Model file for the job. Use its own axes, mm. Face numbers are marked on the shaded views. A direction names the side the tool comes from. Round coordinates to 2 decimals unless told otherwise and drop trailing zeros. Order: outer loops, then holes, each group sorted by start corner. A loop starts at its lowest first (then second) coordinate and runs counter-clockwise, first axis right, second up. Notation, with made-up numbers: (8, -33) -> (64, -33) arc R11 ccw to (64, -14) -> close; hole circle Ø7 at (-5, 13). An arc over 180 degrees is marked (long way). Answer as CSV lines item,"result".
Autodesk Inventor part; units mm, degrees
ref_plane "YZ Plane" through (0, 0, 0) normal (1, 0, 0) x (0, 1, 0)
ref_plane "XZ Plane" through (0, 0, 0) normal (0, 1, 0) x (-1, 0, 0)
ref_plane "XY Plane" through (0, 0, 0) normal (0, 0, 1) x (1, 0, 0)
sketch "Sketch1" plane through (0, 0, 0) normal (0, 0, 1) x (1, 0, 0)
  line L0 (0, 0) -> (25.4, 0)
  line L1 (25.4, 25.4) -> (15.24, 25.4)
  line L2 (15.24, 25.4) -> (15.24, 15.24)
  line L3 (15.24, 15.24) -> (0, 15.24)
  line L4 (0, 15.24) -> (0, 0)
  line L5 (20.32, 25.4) -> (20.32, 0) construction
  circle A0 centre (20.32, 2.75) radius 1.7907
  circle A1 centre (20.32, 19.95) radius 1.7907
  arc A2 (25.4, 15.8417) -> (28.612, 5.828) centre (28.612, 11.35) ccw
  line L6 (40.64, -5.08) -> (25.4, -5.08)
  line L7 (25.4, -5.08) -> (25.4, 0)
  line L8 (25.4, 0) -> (25.4, 6.8583) construction
  line L9 (25.4, 15.8417) -> (25.4, 25.4)
  line L10 (28.612, 5.828) -> (40.64, 5.828)
  line L11 (40.64, 5.828) -> (40.64, -5.08)
  dimension "d0" = 25.4
  dimension "d1" = 25.4
  dimension "d2" = 10.16
  dimension "d3" = 10.16
  dimension "d4" = 3.5814
  dimension "d6" = 2.75
  dimension "d7" = 3.5814
  dimension "d17" = 17.2
  dimension "d18" = 11.044
  dimension "d20" = 11.35
  dimension "d21" = 8.292
  dimension "d24" = 15.24
  dimension "d25" = 5.08
  dimension "d26" = 15.24
extrude "Extrusion1" add sketch "Sketch1" along normal mid plane 6.35
sketch "Sketch2" plane through (0, 15.24, 3.175) normal (0, 1, 0) x (1, 0, 0)
  line L0 (0, 3.175) -> (15.24, 3.175) construction
  line L1 (15.24, 6.35) -> (15.24, 0)
  circle A0 centre (2.54, 3.175) radius 1.4605
  circle A1 centre (12.7, 3.175) radius 1.4605
  line L2 (0, 6.35) -> (0, 0)
  dimension "d11" = 2.921
  dimension "d12" = 2.921
  dimension "d13" = 2.54
  dimension "d14" = 12.7
extrude "Extrusion2" cut sketch "Sketch2" against normal up to next
sketch "Sketch4" plane through (25.4, -5.08, 3.175) normal (0, -1, 0) x (1, 0, 0)
  circle A0 centre (-22.86, -3.175) radius 1.4605
  circle A1 centre (-12.7, -3.175) radius 1.4605
  line L0 (0, -6.35) -> (0, 0)
  line L1 (-25.4, 0) -> (0, 0)
  line L2 (-25.4, 0) -> (-25.4, -6.35)
  line L3 (0, -6.35) -> (-25.4, -6.35)
  line L4 (15.24, -6.35) -> (15.24, 0)
  line L5 (0, 0) -> (15.24, 0)
  line L6 (0, -6.35) -> (0, 0)
  line L7 (15.24, -6.35) -> (0, -6.35)
  point P0 (-25.4, -3.175)
sketch "Sketch5" plane through (0, 0, 3.175) normal (-1, 0, 0) x (0, 0, 1)
  line L0 (0, 0) -> (-6.35, 0)
  line L1 (0, 15.24) -> (0, 0)
  line L2 (-6.35, 15.24) -> (0, 15.24)
  line L3 (-6.35, 0) -> (-6.35, 15.24)
  point P0 (-3.175, 0)
extrude "Extrusion3" add sketch "Sketch5" along normal blind 5.08
sketch "Sketch6" plane through (0, 0, -3.175) normal (0, 0, -1) x (-1, 0, 0)
  circle A0 centre (-20.32, 19.95) radius 1.7907
  circle A1 centre (-20.32, 2.75) radius 1.7907
  line L0 (-25.4, 0) -> (5.08, 0)
  line L1 (5.08, 15.24) -> (5.08, 0)
  line L2 (-15.24, 15.24) -> (5.08, 15.24)
  line L3 (-15.24, 15.24) -> (-15.24, 25.4)
  line L4 (-15.24, 25.4) -> (-25.4, 25.4)
  line L5 (-25.4, 25.4) -> (-25.4, 15.8417)
  arc A2 (-28.612, 5.828) -> (-25.4, 15.8417) centre (-28.612, 11.35) ccw
  line L6 (-28.612, 5.828) -> (-40.64, 5.828)
  line L7 (-40.64, 5.828) -> (-40.64, -5.08)
  line L8 (-40.64, -5.08) -> (-25.4, -5.08)
  line L9 (-25.4, -5.08) -> (-25.4, 0)
  line L10 (-11.2395, 15.24) -> (-11.2395, 0)
  line L11 (-11.2395, 15.24) -> (-11.2395, 0)
  line L12 (-14.1605, 15.24) -> (-11.2395, 15.24)
  line L13 (-14.1605, 15.24) -> (-14.1605, 0)
  line L14 (-25.4, 0) -> (5.08, 0)
  line L15 (-4.0005, 15.24) -> (-1.0795, 15.24)
  line L16 (-1.0795, 15.24) -> (-1.0795, 0)
  line L17 (-4.0005, 15.24) -> (-4.0005, 0)
  line L18 (-4.0005, 15.24) -> (-4.0005, 0)
properties part number "MotorHolder 2"
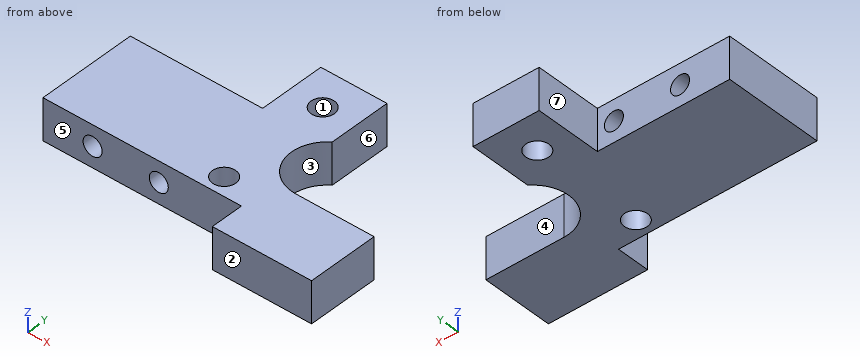
Q1. Saw through at C-C (x = 20.32). Write the cut outline in (y, z) (3 decimals), plus the area to 3 significant figures.
Checks:
outline,"(0, -3.175) -> (0.959, -3.175) -> (0.959, 3.175) -> (0, 3.175) -> close; (4.541, -3.175) -> (18.159, -3.175) -> (18.159, 3.175) -> (4.541, 3.175) -> close; (21.741, -3.175) -> (25.4, -3.175) -> (25.4, 3.175) -> (21.741, 3.175) -> close"
area,"116 mm²"
Q2. Wall check: L1, parallel to Y at x = 20.32, z = 1.25; L2, parallel to X at y = 5.5, z = 0; L3, parallel to X at y = 11, z = 0. Give the ranges that are in metal, low to high. Write a range as [from, to].
Checks:
L1,"[0, 0.96], [4.54, 18.16], [21.74, 25.4]"
L2,"[-5.08, 1.08], [4, 11.24], [14.16, 40.64]"
L3,"[-5.08, 1.08], [4, 11.24], [14.16, 23.1]"
Q3. Saw through at B-B (x = 2.54). Write the cut outline in (y, z) (1 decimal), plus the area to 3 significant figures.
Checks:
outline,"(0, -3.2) -> (15.2, -3.2) -> (15.2, -1.5) -> (0, -1.5) -> close; (0, 1.5) -> (15.2, 1.5) -> (15.2, 3.2) -> (0, 3.2) -> close"
area,"52.3 mm²"
Q4. Mould opens along Y. For the marked faces 1, 2, 3 and 4 say: +Y half, -Y half, draft (parallel to the pull), parting line (faces both ways), or undercut.
Checks:
face 1,"undercut"
face 2,"-Y half"
face 3,"undercut"
face 4,"+Y half"
Q5. Saw through at D-D (z = 2). Write the cut outline in (x, y).
Checks:
outline,"(-5.08, 0) -> (25.4, 0) -> (25.4, -5.08) -> (40.64, -5.08) -> (40.64, 5.83) -> (28.61, 5.83) arc R5.52 cw to (25.4, 15.84) -> (25.4, 25.4) -> (15.24, 25.4) -> (15.24, 15.24) -> (-5.08, 15.24) -> close; hole circle Ø3.58 at (20.32, 2.75); hole circle Ø3.58 at (20.32, 19.95)"
Q6. Tool access for the marked faces 5, 6 and 7: list every direction of +Z, -Z, +X, -X, +Y, -Y with a clear straight run to the whole face (end or side of a thin tool).
Checks:
face 5,"+Z, -Z, -X, -Y"
face 6,"+Z, -Z, +X, +Y"
face 7,"+Z, -Z, -X, +Y"
Q7. Flat gauge pins, fed straight in: pin 1 (1.9 mm diameter, centred on y = 20.5, z = -1, fed in from -X); pin 2 (1.9 mm diameter, centred on x = 5.5, z = 0, fed in from +Y); pin 3 (1.5 mm diameter, centred on y = 22, z = 0, fed in from +X). Where does each tip first touch, or does it go through?
Checks:
pin 1,"x = 15.24"
pin 2,"y = 15.24"
pin 3,"x = 25.4"
Q8. Saw through at A-A (z = 0). Write the cut outline in (x, y).
Checks:
outline,"(-5.08, 0) -> (1.08, 0) -> (1.08, 15.24) -> (-5.08, 15.24) -> close; (4, 0) -> (11.24, 0) -> (11.24, 15.24) -> (4, 15.24) -> close; (14.16, 0) -> (25.4, 0) -> (25.4, -5.08) -> (40.64, -5.08) -> (40.64, 5.83) -> (28.61, 5.83) arc R5.52 cw to (25.4, 15.84) -> (25.4, 25.4) -> (15.24, 25.4) -> (15.24, 15.24) -> (14.16, 15.24) -> close; hole circle Ø3.58 at (20.32, 2.75); hole circle Ø3.58 at (20.32, 19.95)"
